Source: CAD feature listing. Evaluate the final solid. Frame: model axes, mm. Face numbers are marked on the shaded views. A direction names the side the tool comes from. Coordinates: 2 decimals unless noted, no trailing zeros. Write each loop counter-clockwise with the first axis right and the second up, starting at its lowest first coordinate (ties: lowest second). Pieces come first, ordered by that corner, then holes. Notation, with made-up numbers: (-32.75, 12.5) - (5.25, 12.5) arc R19 ccw to (5.25, 41.5) - close; hole circle Ø7 at (-3.5, 19.25). An arc over 180 degrees is marked (long way). One line per question, with ' | ' between items.
from build123d import *

# Parameters (mm, degrees)
PAD_DEPTH = 8


with BuildPart() as part:
    # Sketch → Pad (new body)
    with BuildSketch(Plane.XY):
        with BuildLine():
            Line((-2.5, 30), (37.5, 30))
            Line((37.5, 30), (2.5, 22))
            Line((2.5, 22), (2.5, -30))
            ThreePointArc((-31.5, -29.999997), (-14.500001, -46.999997), (2.5, -30))
            Line((-31.5, -29.999997), (-31.5, -14.999997))
            Line((-31.5, -14.999997), (-26.5, -14.999997))
            Line((-26.5, -14.999997), (-26.5, -29.999997))
            ThreePointArc((-26.5, -29.999997), (-14.500001, -41.999997), (-2.5, -30))
            Line((-2.5, -30), (-2.5, 30))
        make_face()
    extrude(amount=PAD_DEPTH)


solid = part.part
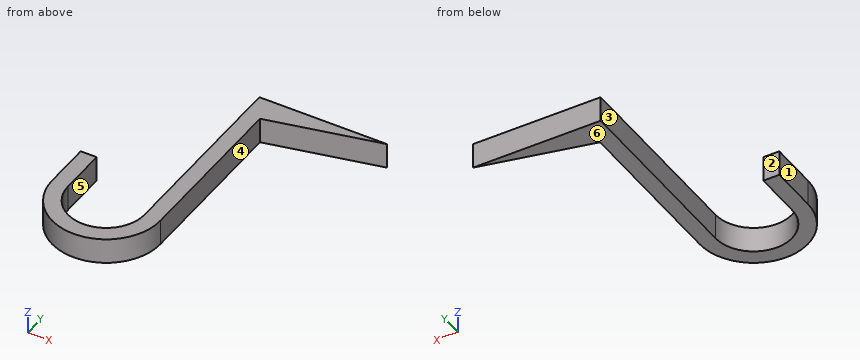
Item 1: Cut plane A-A on y = -28. Return loops of the section in (x, z), and give its area (3 significant figures).
Check sheet entries:
outline: (-31.5, 0) - (-26.5, 0) - (-26.5, 8) - (-31.5, 8) - close; (-2.5, 0) - (2.5, 0) - (2.5, 8) - (-2.5, 8) - close | area: 80.0 mm²
Item 2: Cut plane B-B on z = 1.5. Return loops of the section in (x, y).
Check sheet entries:
outline: (-31.5, -30) arc R17 ccw to (2.5, -30) - (2.5, 22) - (37.5, 30) - (-2.5, 30) - (-2.5, -30) arc R12 cw to (-26.5, -30) - (-26.5, -15) - (-31.5, -15) - close
Item 3: Ray query, line 1 along X through (y, z) = (-19.5, 6.5); line 2 along X through (y, z) = (13, 3.25); line 3 along X through (y, z) = (-35, 2). Return the intervals inside material, ascending. Write a range as [from, to].
Check sheet entries:
line 1: [-31.5, -26.5], [-2.5, 2.5] | line 2: [-2.5, 2.5] | line 3: [-30.75, -25.41], [-3.59, 1.75]
Item 4: Access query for the marked faces 4, 5 and 6. Directions: +Z, -Z, +X, -X, +Y, -Y. A direction counts if a zero-diameter tool reaches every point of the face in a straight line with its end or side. Return the directions, or none.
Check sheet entries:
face 4: +Z, -Z, +X, -Y | face 5: +Z, -Z, +Y | face 6: -Z, +X, -X, +Y, -Y
Item 5: Mould query, pull axis X, two halves, no side actions, for the marked faces 1, 2 and 3. Classes: pulls with the +X half, pulls with the -X half, needs draft (parallel to the pull), parting line crosses it, or undercut.
Check sheet entries:
face 1: pulls with the -X half | face 2: needs draft | face 3: undercut
Item 6: Pin query (flat end, axial travel): pin 1 Ø2.5 at (y, z) = (1, 4.5) entering from +X; pin 2 Ø4 at (y, z) = (17, 6) entering from -X; pin 3 Ø2.5 at (x, z) = (-29, 3.5) entering from +Y. Return the tip coordinate at first contact, or that it passes through.
Check sheet entries:
pin 1: x = 2.5 | pin 2: x = -2.5 | pin 3: y = -15
Item 7: Cut plane D-D on y = -40. Return loops of the section in (x, z).
Check sheet entries:
outline: (-28.25, 0) - (-21.13, 0) - (-21.13, 8) - (-28.25, 8) - close; (-7.87, 0) - (-0.75, 0) - (-0.75, 8) - (-7.87, 8) - close
Item 8: Cut plane C-C on x = -14.5. Return loops of the section in (y, z), and give its area (3 significant figures).
Check sheet entries:
outline: (-47, 0) - (-42, 0) - (-42, 8) - (-47, 8) - close | area: 40.0 mm²
